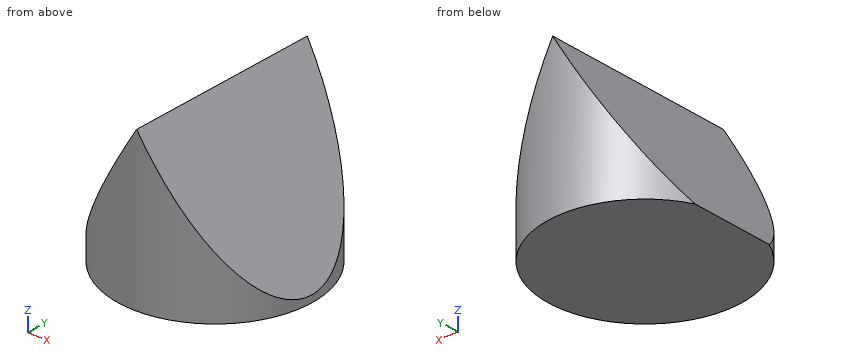
from build123d import *

# Parameters (mm, degrees)
F0_W     = 83.739126
F0_H     = 85.135351
F1_DEPTH = 76.2
F2_W     = 83.739126
F2_H     = 85.135351
F2_R     = 32.565114
F3_DEPTH = 76.2
F4_R     = 86.130148
F5_DEPTH = 152.4


with BuildPart() as f1:
    # F0 (on Top) → F1 (new body)
    with BuildSketch(Plane.XY):
        with Locations((65.940666, 56.417251)):
            Rectangle(F0_W, F0_H)
    extrude(amount=F1_DEPTH)

    # F2 (on face) → F3 (cut)
    with BuildSketch(Plane.XY.offset(76.2)):
        with Locations((65.940666, 56.417251)):
            Rectangle(F2_W, F2_H)
        with Locations((64.77081, 56.190282)):
            Circle(F2_R, mode=Mode.SUBTRACT)
    extrude(amount=-F3_DEPTH, mode=Mode.SUBTRACT)

    # F4 (on Front) → F5 (cut)
    with BuildSketch(Plane.XZ):
        with Locations((64.846843, 15.613325)):
            Circle(F4_R)
        Polygon((98.717026, 0), (35.403937, 0), (67.116521, 52.486237), align=None, mode=Mode.SUBTRACT)
    extrude(amount=-F5_DEPTH, mode=Mode.SUBTRACT)


solid = f1.part
Geometry: final body of the model. Coordinates: model frame, mm. Coordinates: 2 decimals unless noted, no trailing zeros. Order: outer loops, then holes, each group sorted by start corner. A loop starts at its lowest first (then second) coordinate and runs counter-clockwise, first axis right, second up. Notation, with made-up numbers: (37, -34) - (81, -34) arc R19 ccw to (81, -3) - close; hole circle Ø11 at (28, -10). An arc over 180 degrees is marked (long way). Use one line per item in the form item = value.
1) Section C-C (z = 25). Return loops of the section in (x, y), then the cut area to 3 significant figures.
Solutions:
outline = (50.51, 26.91) arc R32.57 ccw to (83.67, 29.67) - (83.67, 82.71) arc R32.57 ccw to (50.51, 85.47) - close
area = 2,060 mm^2
2) Pin query (flat end, axial travel): pin 1 (8 mm diameter, centred on x = 68, z = 40.5, fed in from +Y); pin 2 (12 mm diameter, centred on y = 44.5, z = 44.5, fed in from -X); pin 3 (1 mm diameter, centred on x = 63, y = 75.5, fed in from +Z); pin 4 (8 mm diameter, centred on x = 85.5, y = 65, fed in from -Z). Return the tip coordinate at first contact, or that it passes through.
Solutions:
pin_1 = 88.76
pin_2 = 58.67
pin_3 = 46.5
pin_4 = 0
3) Section B-B (x = 47). Return loops of the section in (y, z), then the cut area to 3 significant figures.
Solutions:
outline = (28.9, 0) - (83.48, 0) - (83.48, 19.19) - (28.9, 19.19) - close
area = 1,050 mm^2
4) Ray query, L1, parallel to Y at x = 56, z = 21.5; L2, parallel to X at y = 73, z = 21; L3, parallel to X at y = 36.5, z = 43. Return the intervals inside material, ascending.
Solutions:
L1 = 24.83 to 87.55
L2 = 48.09 to 86.07
L3 = 61.38 to 72.83
5) Section A-A (y = 28). Return loops of the section in (x, z).
Solutions:
outline = (48.47, 0) - (81.07, 0) - (81.07, 29.3) - (67.12, 52.49) - (48.47, 21.62) - close
6) Section D-D (y = 73). Return loops of the section in (x, z), then the cut area to 3 significant figures.
Solutions:
outline = (36.88, 0) - (92.66, 0) - (92.66, 10.06) - (67.12, 52.49) - (36.88, 2.44) - close
area = 1,630 mm^2
